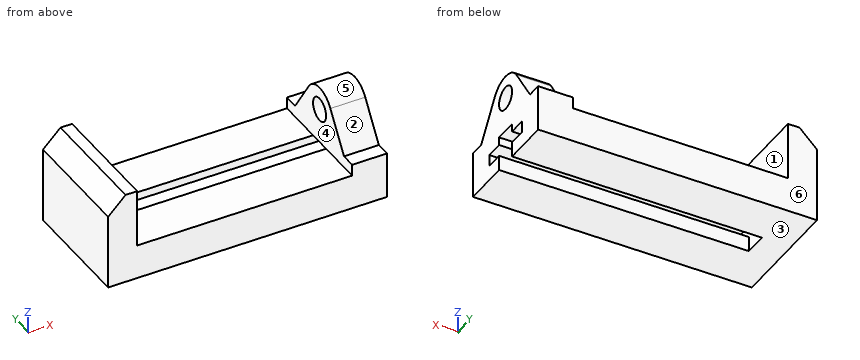
from build123d import *

# Parameters (mm, degrees)
F1_DEPTH = 4.625
F2_R     = 0.5
F3_DEPTH = 1.5
F5_DEPTH = 1.25
F6_SIZE2 = 0.75
F6_SIZE  = 0.75


with BuildPart() as f1:
    # F0 (on Right) → F1 (new body, symmetric)
    with BuildSketch(Plane.YZ):
        Polygon((0, 1.5), (0, 0), (2, 0), (2, 0.65), (1.25, 0.65), (1.25, 1.15), (2, 1.15), (2, 1.5), align=None)
    extrude(amount=F1_DEPTH, both=True)



with BuildPart() as f1b:
    # F0 (on Right) → F1, piece 2 (new body, symmetric)
    with BuildSketch(Plane.YZ):
        Polygon((3, 0.65), (3, 0), (5, 0), (5, 1.5), (3, 1.5), (3, 1.15), (3.75, 1.15), (3.75, 0.65), align=None)
    extrude(amount=F1_DEPTH, both=True)


with BuildPart() as f1_1:
    add(f1.part)

    add(f1b.part)  # F3 merges F1b
    # F2 (on face) → F3 (join)
    with BuildSketch(Plane.YZ.offset(4.625)):
        with BuildLine():
            Line((0, 2), (0, 1.5))
            Line((0, 1.5), (2, 1.5))
            Line((2, 1.5), (3, 1.5))
            Line((3, 1.5), (3, 1.15))
            Line((3, 1.15), (3.75, 1.15))
            Line((3.75, 1.15), (3.75, 0.65))
            Line((3.75, 0.65), (3, 0.65))
            Line((3, 0.65), (3, 0))
            Line((3, 0), (5, 0))
            Line((5, 0), (5, 2))
            Line((5, 2), (4.375, 2))
            Line((4.375, 2), (3.330449827, 3.5570934256))
            ThreePointArc((3.330449827, 3.5570934256), (2.5, 4), (1.669550173, 3.5570934256))
            Line((1.669550173, 3.5570934256), (0.625, 2))
            Line((0.625, 2), (0, 2))
        make_face()
        with Locations((2.5, 3)):
            Circle(F2_R, mode=Mode.SUBTRACT)
        Polygon((0, 1.5), (0, 0), (2, 0), (2, 0.65), (1.25, 0.65), (1.25, 1.15), (2, 1.15), (2, 1.5), align=None)
    extrude(amount=F3_DEPTH)

    # F4 (on face) → F5 (join)
    with BuildSketch(Plane(origin=(-4.625, 0, 0), x_dir=(0, -1, 0), z_dir=(-1, 0, 0))):
        Polygon((-5, 1.5), (-5, 0), (0, 0), (0, 4), (-5, 4), align=None)
    extrude(amount=F5_DEPTH)

    # F6
    f6_edges = [f1_1.edges().sort_by_distance(p)[0] for p in [
        (-5.875, 2.5, 4),
    ]]
    chamfer(f6_edges, length=F6_SIZE, length2=F6_SIZE2)


solid = f1_1.part
For this review, take the finished solid that the model builds, in its own axes (mm). Face numbers are marked on the shaded views. A direction names the side the tool comes from. Coordinates: 2 decimals unless noted, no trailing zeros. Write each loop counter-clockwise with the first axis right and the second up, starting at its lowest first coordinate (ties: lowest second). Pieces come first, ordered by that corner, then holes. Notation, with made-up numbers: (61, -30.75) -> (97, -30.75) arc R7 cw to (97, -23.75) -> close; hole circle Ø9 at (54.5, -30.75). An arc over 180 degrees is marked (long way). Write each question's results on one line, items separated by ' | '. Start each with the question number.
1) Consider section D-D (z = 1.3). Write out the cut boundary in (x, y) (3 decimals), plus the area to 4 significant figures.
2) Consider section C-C (z = 3). Write out the cut boundary in (x, y) (3 decimals), plus the area to 3 significant figures.
3) Wall thickness on L1, parallel to Z at x = 5.2, y = 2.5; L2, parallel to Y at x = -4.5, z = 0.85; L3, parallel to X at y = 4.55, z = 1.75 (3 decimals): over which ranges is each line inside the solid? List them lowest first. Write a range as [from, to].
4) Consider section B-B (x = 1). Write out the cut boundary in (y, z).
5) For the marked faces 4, 5 and 6, list the 3-axis set-ups (+Z, -Z, +X, -X, +Y, -Y) from which the entire face can be reached by the end or side of a thin tool; tool diameter is ignored.
6) Consider section A-A (y = 2.5). Write out the cut boundary in (x, z) (3 decimals).
7) The part is to be moulded in two halves that separate along Y. For the marked faces 1, 2 and 3, say which applies: +Y half, -Y half, draft (parallel to the pull), parting line (faces both ways), or undercut.
8) Insertion check: pin 1 (1 mm diameter, centred on x = -1.5, y = 1.5, fed in from +Z); pin 2 (1 mm diameter, centred on x = 4.5, z = 3, fed in from +Y); pin 3 (0.5 mm diameter, centred on x = 5.5, y = 0.5, fed in from +Z). Each pin has a flat end and moves straight along its axis. Give the tip position at first contact, or say it passes through.
Geometry says:
1) outline: (-5.875, 0) -> (6.125, 0) -> (6.125, 2) -> (-4.625, 2) -> (-4.625, 3) -> (6.125, 3) -> (6.125, 5) -> (-5.875, 5) -> close | area: 49.25 mm^2
2) outline: (-5.875, 0) -> (-4.625, 0) -> (-4.625, 5) -> (-5.875, 5) -> close; (4.625, 1.296) -> (6.125, 1.296) -> (6.125, 2) -> (4.625, 2) -> close; (4.625, 3) -> (6.125, 3) -> (6.125, 3.704) -> (4.625, 3.704) -> close | area: 8.36 mm^2
3) L1: [1.5, 2.5], [3.5, 4] | L2: [0, 1.25], [3.75, 5] | L3: [-5.875, -4.625], [4.625, 6.125]
4) outline: (0, 0) -> (2, 0) -> (2, 0.65) -> (1.25, 0.65) -> (1.25, 1.15) -> (2, 1.15) -> (2, 1.5) -> (0, 1.5) -> close; (3, 0) -> (5, 0) -> (5, 1.5) -> (3, 1.5) -> (3, 1.15) -> (3.75, 1.15) -> (3.75, 0.65) -> (3, 0.65) -> close
5) face 4: +Z, +Y, -Y | face 5: +Z, +X | face 6: +Z, -Z, +X, -X, +Y
6) outline: (-5.875, 0) -> (-4.625, 0) -> (-4.625, 4) -> (-5.125, 4) -> (-5.875, 3.25) -> close; (4.625, 1.5) -> (6.125, 1.5) -> (6.125, 2.5) -> (4.625, 2.5) -> close; (4.625, 3.5) -> (6.125, 3.5) -> (6.125, 4) -> (4.625, 4) -> close
7) face 1: undercut | face 2: -Y half | face 3: draft
8) pin 1: z = 1.5 | pin 2: y = 4.03 | pin 3: z = 2.19
